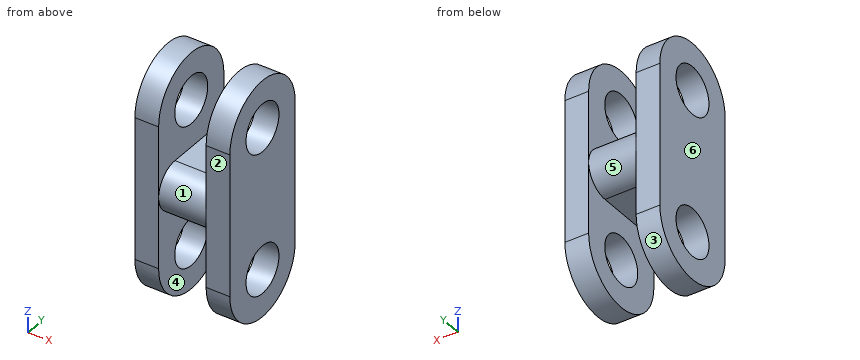
```python
from build123d import *

# Parameters (mm, degrees)
BOSS_EXTRUDE1_DEPTH = 2.5
BOSS_EXTRUDE2_DEPTH = 5
BOSS_EXTRUDE3_DEPTH = 2.5
HOLE1_D             = 5.05
HOLE1_DEPTH         = 2.5
HOLE2_D             = 5.05
HOLE2_DEPTH         = 2.5
HOLE3_D             = 5.05
HOLE3_DEPTH         = 10


with BuildPart() as part:
    # Sketch1 → Boss-Extrude1 (new body)
    with BuildSketch(Plane(origin=(0, 0, 0), x_dir=(0, -1, 0), z_dir=(-1, 0, 0))):
        with BuildLine():
            Line((0, 20), (0, 5))
            ThreePointArc((0, 5), (5, 0), (10, 5))
            Line((10, 5), (10, 20))
            ThreePointArc((10, 20), (5, 25), (0, 20))
        make_face()
    extrude(amount=-BOSS_EXTRUDE1_DEPTH)

    # Sketch2 → Boss-Extrude2 (add)
    with BuildSketch(Plane(origin=(2.5, 0, 0), x_dir=(0, 0, -1), z_dir=(1, 0, 0))):
        with BuildLine():
            Line((-15, -7.5), (-15, -2.5))
            ThreePointArc((-15, -2.5), (-12.5, 0), (-10, -2.5))
            Line((-10, -2.5), (-10, -7.5))
            ThreePointArc((-10, -7.5), (-12.5, -10), (-15, -7.5))
        make_face()
    extrude(amount=BOSS_EXTRUDE2_DEPTH)

    # Sketch3 → Boss-Extrude3 (add)
    with BuildSketch(Plane(origin=(7.5, 0, 0), x_dir=(0, 0, -1), z_dir=(1, 0, 0))):
        with BuildLine():
            Line((-20, 0), (-5, 0))
            ThreePointArc((-5, 0), (0, -5), (-5, -10))
            Line((-5, -10), (-20, -10))
            ThreePointArc((-20, -10), (-25, -5), (-20, 0))
        make_face()
    extrude(amount=BOSS_EXTRUDE3_DEPTH)

    # Hole1
    with Locations(Plane(origin=(10, 0, 0), x_dir=(0, 0, -1), z_dir=(1, 0, 0))):
        with Locations((-5, -5)):
            Hole(HOLE1_D / 2, depth=HOLE1_DEPTH)

    # Hole2
    with Locations(Plane.ZY.offset(-7.5)):
        with Locations((20, -5)):
            Hole(HOLE2_D / 2, depth=HOLE2_DEPTH)

    # Hole3
    with Locations(Plane.ZY):
        with Locations((20, -5), (5, -5)):
            Hole(HOLE3_D / 2, depth=HOLE3_DEPTH)


solid = part.part
```
Check sheet for the modelled part. Datum: model origin and axes. Units: mm. Face numbers are marked on the shaded views. A direction names the side the tool comes from. Give positions to 0.01 mm unless a question says otherwise; leave off trailing zeros. Order: outer loops, then holes, each group sorted by start corner. A loop starts at its lowest first (then second) coordinate and runs counter-clockwise, first axis right, second up. Notation, with made-up numbers: (34.25, 42) -> (69.25, 42) arc R31 cw to (69.25, 81) -> close; hole circle Ø8 at (8.5, -24.5). An arc over 180 degrees is marked (long way). Use CSV: the item, a comma, the result in double quotes. Start each with the question number.
1) Set-up check for the marked faces 1 and 2: record each of +Z, -Z, +X, -X, +Y, -Y from which the full face is reachable in a straight line by a thin tool's end or side.
2) Sectioned sample at A-A, the plane y = -5. Record the boundary of the cut face in (x, z) (3 decimals).
3) Sectioned sample at B-B, the plane z = 17.75. Record the boundary of the cut face in (x, y), plus the area to 3 significant figures.
4) Go/stop test with flat-tipped pins: P1, Ø2.5, axis at x = 5.5, y = -5.5, coming from the -Z side; P2, Ø2.5, axis at x = 6, y = -5, coming from the +Z side. Record where each tip stops, or that it passes through.
5) Material ranges on line 1 (X direction, y = -8, z = 16.25); line 2 (Y direction, x = 1.1, z = 20) (3 decimals); line 3 (Z direction, x = 1.75, y = -7), recorded low to high. Write a range as from..to.
6) Sectioned sample at D-D, the plane y = -8.5. Record the boundary of the cut face in (x, z), plus the area to 3 significant figures.
7) Mould release check, pull along X, two halves, no side actions. Record for the marked faces 3, 4, 5 and 6: released by +X, released by -X, zero draft, split by the parting line, or undercut.
8) Sectioned sample at C-C, the plane x = 1.5. Record the boundary of the cut face in (y, z) (3 decimals), plus the area to 3 significant figures.
Recorded:
1,face 1,"-Y"
1,face 2,"+Z, -Z, +X, -X, -Y"
2,outline,"(0, 0) -> (2.5, 0) -> (2.5, 2.475) -> (0, 2.475) -> close; (0, 7.525) -> (2.5, 7.525) -> (2.5, 10) -> (7.5, 10) -> (7.5, 7.525) -> (10, 7.525) -> (10, 17.475) -> (7.5, 17.475) -> (7.5, 15) -> (2.5, 15) -> (2.5, 17.475) -> (0, 17.475) -> close; (0, 22.525) -> (2.5, 22.525) -> (2.5, 25) -> (0, 25) -> close; (7.5, 0) -> (10, 0) -> (10, 2.475) -> (7.5, 2.475) -> close; (7.5, 22.525) -> (10, 22.525) -> (10, 25) -> (7.5, 25) -> close"
3,outline,"(0, -10) -> (2.5, -10) -> (2.5, -6.15) -> (0, -6.15) -> close; (0, -3.85) -> (2.5, -3.85) -> (2.5, 0) -> (0, 0) -> close; (7.5, -10) -> (10, -10) -> (10, -6.15) -> (7.5, -6.15) -> close; (7.5, -3.85) -> (10, -3.85) -> (10, 0) -> (7.5, 0) -> close"
3,area,"38.5 mm2"
4,P1,"z = 10"
4,P2,"z = 15"
5,line 1,"0..2.5, 7.5..10"
5,line 2,"-10..-7.525, -2.475..0"
5,line 3,"0.42..3.46, 6.54..18.46, 21.54..24.58"
6,outline,"(0, 1.43) -> (2.5, 1.43) -> (2.5, 10.21) -> (7.5, 10.21) -> (7.5, 1.43) -> (10, 1.43) -> (10, 23.57) -> (7.5, 23.57) -> (7.5, 14.79) -> (2.5, 14.79) -> (2.5, 23.57) -> (0, 23.57) -> close"
6,area,"134 mm2"
7,face 3,"zero draft"
7,face 4,"undercut"
7,face 5,"undercut"
7,face 6,"released by -X"
8,outline,"(-10, 5) arc R5 ccw to (0, 5) -> (0, 20) arc R5 ccw to (-10, 20) -> close; hole circle Ø5.05 at (-5, 5); hole circle Ø5.05 at (-5, 20)"
8,area,"188 mm2"
